Can you work these out from the model? Positions are in its coordinate system, mm. Face numbers are marked on the shaded views. A direction names the side the tool comes from. Give positions to 0.01 mm unless a question says otherwise; leave off trailing zeros. Write each loop counter-clockwise with the first axis right and the second up, starting at its lowest first coordinate (ties: lowest second). Pieces come first, ordered by that corner, then holes.
```python
from build123d import *

# Parameters (mm, degrees)
SKETCH1_W           = 288
SKETCH1_H           = 230
SKETCH1_W_2         = 258
SKETCH1_H_2         = 200
WALLS_DEPTH         = 51
SKETCH3_W           = 288
SKETCH3_H           = 230
BASE_DEPTH          = 15
SKETCH4_W           = 12
SKETCH4_H           = 15.1
LONG_SUPPORT_DEPTH  = 114.5
SKETCH5_W           = 12
SKETCH5_H           = 15.1
SHORT_SUPPORT_DEPTH = 25
CUT_EXTRUDE4_REACH  = 353.219
SKETCH6_R           = 6.35


with BuildPart() as part:
    # Sketch1 → Walls (new body)
    with BuildSketch(Plane(origin=(0, 0, 0), x_dir=(1, 0, 0), z_dir=(0, 1, 0))):
        with Locations((129, 100)):
            Rectangle(SKETCH1_W, SKETCH1_H)
        with Locations((129, 100)):
            Rectangle(SKETCH1_W_2, SKETCH1_H_2, mode=Mode.SUBTRACT)
    extrude(amount=WALLS_DEPTH)

    # Sketch3 → Base (add)
    with BuildSketch(Plane.XZ):
        with Locations((129, -100)):
            Rectangle(SKETCH3_W, SKETCH3_H)
    extrude(amount=BASE_DEPTH)

    # Sketch4 → Long_Support (add, symmetric)
    with BuildSketch(Plane(origin=(129, 0, 0), x_dir=(0, 0, -1), z_dir=(1, 0, 0))):
        with Locations((6, 42.45)):
            Rectangle(SKETCH4_W, SKETCH4_H)
        with Locations((194, 42.45)):
            Rectangle(SKETCH4_W, SKETCH4_H)
    extrude(amount=LONG_SUPPORT_DEPTH, both=True)

    # Sketch5 → Short_Support (add, symmetric)
    with BuildSketch(Plane(origin=(0, 0, -100), x_dir=(-1, 0, 0), z_dir=(0, 0, -1))):
        with Locations((-252, 42.45)):
            Rectangle(SKETCH5_W, SKETCH5_H)
        with Locations((-6, 42.45)):
            Rectangle(SKETCH5_W, SKETCH5_H)
    extrude(amount=SHORT_SUPPORT_DEPTH, both=True)

    # Sketch6 → Cut-Extrude4 (cut, up to next)
    with BuildSketch(Plane(origin=(0, 0, 0), x_dir=(0, 0, -1), z_dir=(1, 0, 0)), mode=Mode.PRIVATE) as cut_extrude4_sk1:
        with Locations((168.65, 43.65)):
            Circle(SKETCH6_R)
    cut_extrude4_tool1 = extrude(cut_extrude4_sk1.sketch, amount=-CUT_EXTRUDE4_REACH, mode=Mode.PRIVATE) & part.part
    add(cut_extrude4_tool1.solids().sort_by_distance((0, 43.65, -168.65))[0], mode=Mode.SUBTRACT)


solid = part.part
```
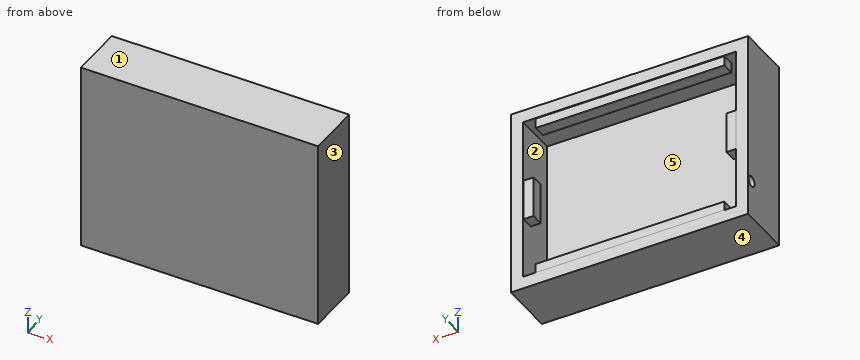
1) Suppose I cut it at B-B on y = 43.65. Write out the boundary of the cut face in (x, z), plus the area to 3 significant figures.
Values follow:
outline: (-15, -215) - (273, -215) - (273, 15) - (-15, 15) - (-15, -162.3) - (0, -162.3) - (0, -125) - (12, -125) - (12, -75) - (0, -75) - (0, 0) - (14.5, 0) - (14.5, -12) - (243.5, -12) - (243.5, 0) - (258, 0) - (258, -75) - (246, -75) - (246, -125) - (258, -125) - (258, -200) - (243.5, -200) - (243.5, -188) - (14.5, -188) - (14.5, -200) - (0, -200) - (0, -175) - (-15, -175) - close
area: 21,100 mm2
2) For the marked faces 1 and 2, which set-ups out of +Z, -Z, +X, -X, +Y, -Y let a thin tool reach every point of the face, with its end or its side?
Values follow:
face 1: +Z, +X, -X, +Y, -Y
face 2: none
3) Suppose I cut it at A-A on z = -168.65. Write out the boundary of the cut face in (x, y), plus the area to 3 significant figures.
Values follow:
outline: (-15, -15) - (273, -15) - (273, 51) - (258, 51) - (258, 0) - (0, 0) - (0, 37.3) - (-15, 37.3) - close; (-15, 50) - (0, 50) - (0, 51) - (-15, 51) - close
area: 5,660 mm2
4) Suppose I cut it at C-C on z = -134. Write out the boundary of the cut face in (x, y), plus the area to 3 significant figures.
Values follow:
outline: (-15, -15) - (273, -15) - (273, 51) - (258, 51) - (258, 0) - (0, 0) - (0, 51) - (-15, 51) - close
area: 5,850 mm2
5) Please list where these lines run through material, in increasing order: L1, parallel to Y at x = -6.5, z = -168.65; L2, parallel to Z at x = -10, y = 43; L3, parallel to Y at x = 93.5, z = -5.
Values follow:
L1: y = -15 to 37.3, 50 to 51
L2: z = -215 to -174.97, -162.33 to 15
L3: y = -15 to 0, 34.9 to 50
6) If we mould it in two halves opening along Z, with no side actions, what happens to the marked faces 3, 4 and 5? For each: +Z half, -Z half, draft (parallel to the pull), parting line (faces both ways), or undercut.
Values follow:
face 3: draft
face 4: -Z half
face 5: undercut
7) For pin 1 Ø3 at (x, z) = (177, -164.5) entering from +Y; pin 2 Ø6 at (x, z) = (7, -107.5) entering from +Y, each with a flat end and sliding along its axis, tell me the tip position at first contact or that it passes through.
Values follow:
pin 1: stops at y = 0
pin 2: stops at y = 50
8) Suppose I cut it at D-D on y = 3.5. Write out the boundary of the cut face in (x, z), plus the area to 3 significant figures.
Values follow:
outline: (-15, -215) - (273, -215) - (273, 15) - (-15, 15) - close; hole (0, -200) - (258, -200) - (258, 0) - (0, 0) - close
area: 14,600 mm2
